```python
from build123d import *

# Parameters (mm, degrees)
BOSS_EXTRUDE4_DEPTH      = 16
BOSS_EXTRUDE4_DEPTH_BACK = 0.625401596
SKETCH2_R                = 4
SKETCH4_R                = 6
BOSS_EXTRUDE5_DEPTH      = 2
SKETCH5_R                = 3
CUT_EXTRUDE1_DEPTH       = 16


with BuildPart() as part:
    # Sketch2 → Boss-Extrude4 (new, two sides: drawn at the far end of the back side and taken through both)
    with BuildSketch(Plane.XY.offset(-BOSS_EXTRUDE4_DEPTH_BACK)):
        Circle(SKETCH2_R)
    extrude(amount=BOSS_EXTRUDE4_DEPTH + BOSS_EXTRUDE4_DEPTH_BACK)

    # Sketch4 → Boss-Extrude5 (add)
    with BuildSketch(Plane.XY.offset(16)):
        Circle(SKETCH4_R)
    extrude(amount=BOSS_EXTRUDE5_DEPTH)

    # Sketch5 → Cut-Extrude1 (cut)
    with BuildSketch(Plane(origin=(0, 0, -0.625401596), x_dir=(-1, 0, 0), z_dir=(0, 0, -1))):
        Circle(SKETCH5_R)
    extrude(amount=-CUT_EXTRUDE1_DEPTH, mode=Mode.SUBTRACT)


solid = part.part
```
Work out the finished part from the listing and answer in its coordinate system (mm). A direction names the side the tool comes from. Round coordinates to 2 decimals unless told otherwise and drop trailing zeros. Order: outer loops, then holes, each group sorted by start corner. A loop starts at its lowest first (then second) coordinate and runs counter-clockwise, first axis right, second up.
Q1. The mould has two halves that part along X. Classify faces 1 (the flat face through (1, 3, -0.625)), 2 (the cylindrical face through (-6, 0, 17)), 3 (the flat face through (0, 0, 15.375)): pulls with the +X half, pulls with the -X half, needs draft (parallel to the pull), parting line crosses it, or undercut.
Solution:
face 1: needs draft
face 2: parting line crosses it
face 3: undercut
Q2. A cutting plane is placed at C-C, the plane z = 10.25. Determine the outline of the cut face in (x, y).
Solution:
outline: circle Ø8 at (0, 0); hole circle Ø6 at (0, 0)
Q3. A tool of negligible diameter and unlimited length cuts with its end or side. For faces 4 (the flat face through (-1.42, -3.92, 16)), 5 (the flat face through (0, 0, 18)), from which of +Z, -Z, +X, -X, +Y, -Y can it reach the whole face along a straight path? Write none if from no direction.
Solution:
face 4: -Z
face 5: +Z, +X, -X, +Y, -Y
Q4. A cutting plane is placed at D-D, the plane z = 16.25. Determine the outline of the cut face in (x, y).
Solution:
outline: circle Ø12 at (0, 0)
Q5. A cutting plane is placed at A-A, the plane x = 0. Determine the outline of the cut face in (y, z), then the cut area to 3 significant figures.
Solution:
outline: (-6, 16) - (-4, 16) - (-4, -0.63) - (-3, -0.63) - (-3, 15.37) - (3, 15.37) - (3, -0.63) - (4, -0.63) - (4, 16) - (6, 16) - (6, 18) - (-6, 18) - close
area: 61.0 mm2
Q6. Find the intervals of material crossed by line 1 along Y through (x, z) = (0, 9.75); line 2 along Z through (x, y) = (-0.5, -4.25); line 3 along Z through (x, y) = (0.5, 1.5), in increasing order.
Solution:
line 1: y = -4 to -3, 3 to 4
line 2: z = 16 to 18
line 3: z = 15.37 to 18
Q7. Given pin 1 Ø2 at (y, z) = (0, 6.5) entering from -X; pin 2 Ø2 at (y, z) = (3, 16) entering from +X, each flat-ended and moving along its own axis, determine where each tip first touches the part or whether it passes through.
Solution:
pin 1: stops at x = -4
pin 2: stops at x = 5.66
